Check sheet for the drawn part. Datum: minimum x, y, z corner. Units: mm. A direction names the side the tool comes from. Give positions to 0.01 mm unless a question says otherwise; leave off trailing zeros. Loops run counter-clockwise (first coordinate to the right, second up) from the corner with the lowest first, then second, coordinate; pieces in that order, holes last.
1. Go/stop test with flat-tipped pins: pin 1 Ø2 at (x, y) = (3.5, 17.5) entering from -Z; pin 2 Ø3 at (x, z) = (5.5, 12) entering from +Y; pin 3 Ø3 at (x, y) = (3.5, 15) entering from +Z (1 decimal). Record where each tip stops, or that it passes through.
2. Tool access check on the marked faces 4, 5, 6 and 7. Record the directions out of +Z, -Z, +X, -X, +Y, -Y that give a thin tool (end or side, any length) a straight path to the whole face; none if there is none.
3. Cross-section at B-B, the plane x = 5.5. Record the cut outline in (y, z), plus the area to 3 significant figures.
4. Cross-section at C-C, the plane x = 1. Record the cut outline in (y, z) (1 decimal).
5. Material ranges on L1, parallel to Y at x = 5, z = 10.5 (1 decimal); L2, parallel to Z at x = 2, y = 13.25 (1 decimal); L3, parallel to Y at x = 0.5, z = 10.75 (1 decimal), recorded low to high.
6. Cross-section at A-A, the plane z = 10.16. Record the cut outline in (x, y) (1 decimal).
7. Release check for a two-part mould opening along Y. For the marked faces 1, 2 and 3 record: +Y half, -Y half, draft (parallel to the pull), parting line (faces both ways), or undercut.
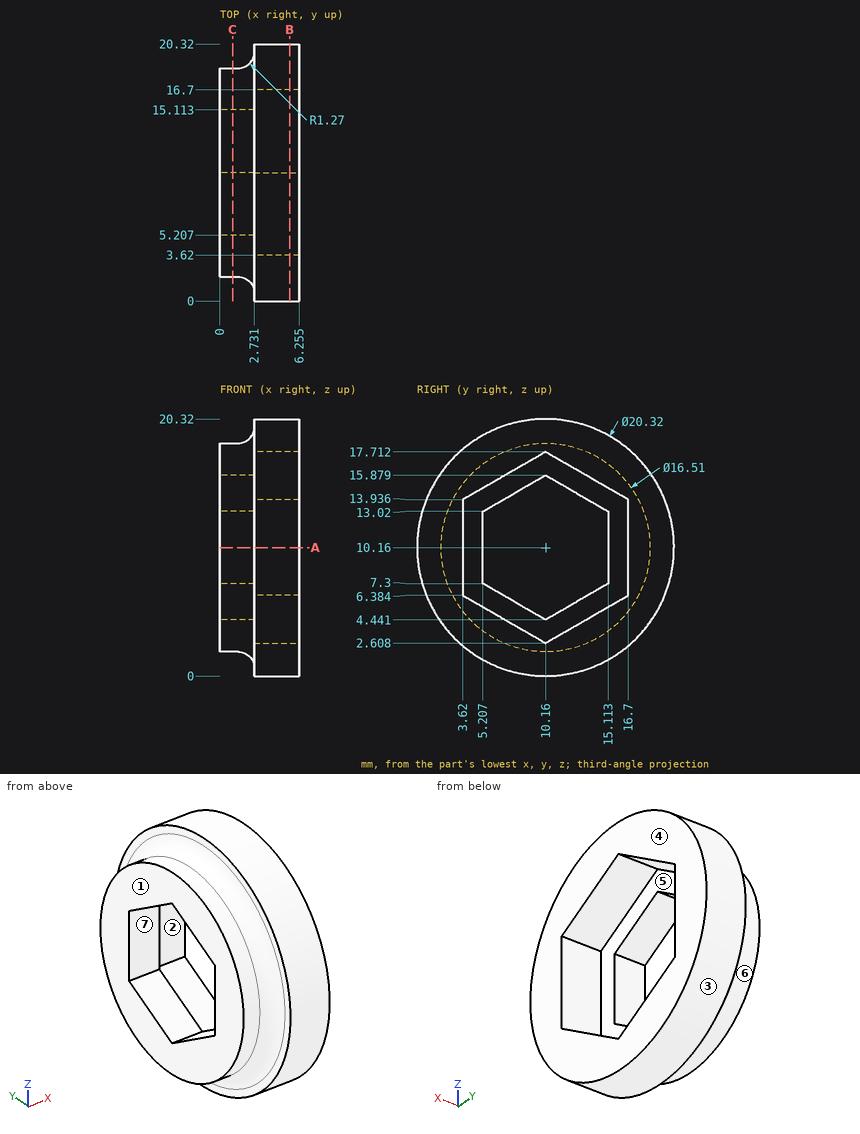
Result:
1. pin 1: stops at z = 2.22
1. pin 2: stops at y = 20.31
1. pin 3: stops at z = 19.8
2. face 4: +Z, -Z, +X, +Y, -Y
2. face 5: +X
2. face 6: -X
2. face 7: +X, -X
3. outline: circle Ø20.32 at (10.16, 10.16); hole (3.62, 6.38) - (10.16, 2.61) - (16.7, 6.38) - (16.7, 13.94) - (10.16, 17.71) - (3.62, 13.94) - close
3. area: 176 mm2
4. outline: circle Ø16.5 at (10.2, 10.2); hole (5.2, 7.3) - (10.2, 4.4) - (15.1, 7.3) - (15.1, 13) - (10.2, 15.9) - (5.2, 13) - close
5. L1: y = 0 to 3.6, 16.7 to 20.3
5. L2: z = 2.4 to 6.2, 14.1 to 17.9
5. L3: y = 1.9 to 5.2, 15.1 to 18.4
6. outline: (0, 1.9) - (1.5, 1.9) arc R1.3 cw to (2.7, 0.6) - (2.7, 0) - (6.3, 0) - (6.3, 3.6) - (2.7, 3.6) - (2.7, 5.2) - (0, 5.2) - close; (0, 15.1) - (2.7, 15.1) - (2.7, 16.7) - (6.3, 16.7) - (6.3, 20.3) - (2.7, 20.3) - (2.7, 19.7) arc R1.3 cw to (1.5, 18.4) - (0, 18.4) - close
7. face 1: draft
7. face 2: undercut
7. face 3: parting line
